CAD build for the part. Positions are in the model's coordinates, mm. Face numbers are marked on the shaded views. Give positions to 0.01 mm unless a question says otherwise; leave off trailing zeros. Order: outer loops, then holes, each group sorted by start corner. A loop starts at its lowest first (then second) coordinate and runs counter-clockwise, first axis right, second up. Notation, with made-up numbers: (-25.5, 4.25) -> (9.5, 4.25) arc R15 cw to (9.5, 32.25) -> close; hole circle Ø7 at (64, 82). An arc over 180 degrees is marked (long way). Use one line per item in the form item = value. Start each with the question number.
1) Cut at A-A, the plane z = -0.5. State how many separate pieces and enclosed holes the cut face has, and give its area (3 significant figures).
2) Probe line 1 (X direction, y = 4.5, z = -4.5); line 2 (X direction, y = -9, z = 1); line 3 (Y direction, x = 1, z = 2.5). List the from-to ranges inside material, lowest first.
3) Cut at B-B, the plane y = -22. Give the cut face in (x, z), and give its area (3 significant figures).
4) Drop flat-ended pins along their axis: P1, Ø2, axis at x = -36, z = 2.5, coming from the -Y side; P2, Ø5, axis at x = -9.5, z = -1.5, coming from the +Y side; P3, Ø4, axis at y = -11, z = -2.5, coming from the -X side. Give the stop position or say it passes through.
5) Cut at D-D, the plane x = 0. Give the cut face in (y, z).
6) Cut at C-C, the plane y = 29. Give the cut face in (x, z), and give its area (3 significant figures).
7) Mould opens along X. For the marked faces 1, 2 and 3 say: pulls with the +X half, pulls with the -X half, needs draft (parallel to the pull), parting line crosses it, or undercut.
from build123d import *

# Parameters (mm, degrees)
SKETCH1_R           = 5
SKETCH1_R_2         = 2
BOSS_EXTRUDE1_DEPTH = 4.75
CUT_EXTRUDE1_DEPTH  = 2


with BuildPart() as part:
    # Sketch1 → Boss-Extrude1 (new, symmetric)
    with BuildSketch(Plane.XY):
        with BuildLine():
            Line((-22.308767332, -29.181670657), (35.698943118, -31.988315456))
            ThreePointArc((35.698943118, -31.988315456), (42.1516901, -30.02280497), (45.888257007, -24.406823948))
            ThreePointArc((45.888257007, -24.406823948), (48.128157677, 1.060560267), (42.475146865, 25.993435805))
            ThreePointArc((42.475146865, 25.993435805), (38.797626972, 30.574489653), (33.182217728, 32.3))
            Line((33.182217728, 32.3), (-34.397529085, 32.3))
            ThreePointArc((-34.397529085, 32.3), (-49.622555092, 34.67439152), (-63.401574193, 41.572056677))
            ThreePointArc((-63.401574193, 41.572056677), (-76.799263642, 49.225759558), (-91.448521696, 54.071013816))
            ThreePointArc((-91.448521696, 54.071013816), (-97.990041102, 53.309279516), (-102.639296293, 48.644931604))
            Line((-102.639296293, 48.644931604), (-123.129936653, 6.033713582))
            ThreePointArc((-123.129936653, 6.033713582), (-120.252485213, -6.197177966), (-107.689906175, -5.960444431))
            Line((-107.689906175, -5.960444431), (-72.864818345, 23.261273923))
            ThreePointArc((-72.864818345, 23.261273923), (-64.470178387, 25.908093735), (-56.662687309, 21.843771132))
            ThreePointArc((-56.662687309, 21.843771132), (-46.805355693, 6.125218695), (-41.605017691, -11.684788659))
            ThreePointArc((-41.605017691, -11.684788659), (-35.091884298, -23.890622031), (-22.308767332, -29.181670657))
        make_face()
        Circle(SKETCH1_R, mode=Mode.SUBTRACT)
        with Locations((36.182217728, -22)):
            Circle(SKETCH1_R_2, mode=Mode.SUBTRACT)
        with Locations((-21.317782272, -8.7)):
            Circle(SKETCH1_R_2, mode=Mode.SUBTRACT)
        with Locations((38.182217728, -0.1)):
            Circle(SKETCH1_R_2, mode=Mode.SUBTRACT)
        with Locations((33.182217728, 22.3)):
            Circle(SKETCH1_R_2, mode=Mode.SUBTRACT)
        with Locations((-31.817782272, 8.3)):
            Circle(SKETCH1_R_2, mode=Mode.SUBTRACT)
        with Locations((-105.317782272, 20)):
            Circle(SKETCH1_R_2, mode=Mode.SUBTRACT)
        with Locations((-114.117782272, 1.7)):
            Circle(SKETCH1_R_2, mode=Mode.SUBTRACT)
    extrude(amount=BOSS_EXTRUDE1_DEPTH, both=True)

    # Sketch2 → Cut-Extrude1 (cut, symmetric)
    with BuildSketch(Plane.XY):
        with BuildLine():
            Line((-78.227129447, 18.761760655), (-91.668909505, 44.876871439))
            Line((-91.668909505, 44.876871439), (-92.486661389, 54.245970368))
            ThreePointArc((-92.486661389, 54.245970368), (-96.402275052, 53.918435936), (-99.889427329, 52.10761343))
            Line((-99.889427329, 52.10761343), (-95.58537432, 43.745564604))
            Line((-95.58537432, 43.745564604), (-92.369017313, 6.895307763))
            Line((-92.369017313, 6.895307763), (-78.227129447, 18.761760655))
        make_face()
    extrude(amount=CUT_EXTRUDE1_DEPTH, both=True, mode=Mode.SUBTRACT)


solid = part.part
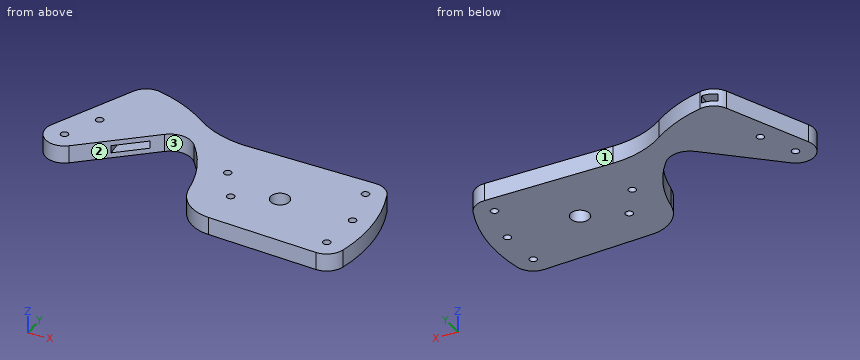
Result:
q1.separate_pieces = 2
q1.enclosed_holes = 8
q1.area = 7,420 mm²
q2.line_1 = -123.72 to -95.22, -46.1 to -2.18, 2.18 to 47.82
q2.line_2 = -42.06 to -23.3, -19.34 to 48.2
q2.line_3 = -30.31 to -4.9, 4.9 to 32.3
q3.outline = (-36.93, -4.75) -> (34.18, -4.75) -> (34.18, 4.75) -> (-36.93, 4.75) -> close; (38.18, -4.75) -> (46.45, -4.75) -> (46.45, 4.75) -> (38.18, 4.75) -> close
q3.area = 754 mm²
q4.P1 = -23.97
q4.P2 = 32.3
q4.P3 = -42.06
q5.outline = (-30.26, -4.75) -> (-5, -4.75) -> (-5, 4.75) -> (-30.26, 4.75) -> close; (5, -4.75) -> (32.3, -4.75) -> (32.3, 4.75) -> (5, 4.75) -> close
q6.outline = (-112.09, -4.75) -> (40.61, -4.75) -> (40.61, 4.75) -> (-112.09, 4.75) -> close; hole (-94.3, -2) -> (-83.5, -2) -> (-83.5, 2) -> (-94.3, 2) -> close
q6.area = 1,410 mm²
q7.face_1 = needs draft
q7.face_2 = undercut
q7.face_3 = undercut
